```python
from build123d import *

# Parameters (mm, degrees)
SKETCH1_W                = 346
SKETCH1_H                = 134.5
BOSS_EXTRUDE1_DEPTH      = 6
M5_CLEARANCE_HOLE1_D     = 5.3
M5_CLEARANCE_HOLE2_D     = 5.3
SKETCH5_W                = 140
SKETCH5_H                = 70.4
CUT_EXTRUDE1_DEPTH       = 7
SKETCH6_R                = 10
BOSS_EXTRUDE2_DEPTH      = 6
FILLET1_R                = 5
M2_5_CLEARANCE_HOLE1_D   = 2.7
CUT_EXTRUDE29_DEPTH      = 7
SKETCH72_W               = 6.1
SKETCH72_H               = 10.1
CUT_EXTRUDE2_DEPTH       = 4
CUT_EXTRUDE2_DEPTH_BACK  = 4
SKETCH73_W               = 6.1
SKETCH73_H               = 10.1
CUT_EXTRUDE21_DEPTH      = 4
CUT_EXTRUDE21_DEPTH_BACK = 4
SKETCH74_W               = 6.1
SKETCH74_H               = 10.1
CUT_EXTRUDE22_DEPTH      = 4
CUT_EXTRUDE22_DEPTH_BACK = 4
SKETCH75_W               = 6.1
SKETCH75_H               = 10.1
CUT_EXTRUDE23_DEPTH      = 4
CUT_EXTRUDE23_DEPTH_BACK = 4
SKETCH76_W               = 6.1
SKETCH76_H               = 10.1
CUT_EXTRUDE24_DEPTH      = 4
CUT_EXTRUDE24_DEPTH_BACK = 4
SKETCH771_W              = 6.1
SKETCH771_H              = 10.1
CUT_EXTRUDE25_DEPTH      = 4
CUT_EXTRUDE25_DEPTH_BACK = 4
SKETCH781_W              = 6.1
SKETCH781_H              = 10.1
CUT_EXTRUDE26_DEPTH      = 4
CUT_EXTRUDE26_DEPTH_BACK = 4
SKETCH79_W               = 6.1
SKETCH79_H               = 10.1
CUT_EXTRUDE27_DEPTH      = 4
CUT_EXTRUDE27_DEPTH_BACK = 4
SKETCH710_W              = 6.1
SKETCH710_H              = 10.1
CUT_EXTRUDE28_DEPTH      = 4
CUT_EXTRUDE28_DEPTH_BACK = 4
SKETCH63_W               = 10
SKETCH63_H               = 6
CUT_EXTRUDE13_DEPTH      = 4
SKETCH64_W               = 10
SKETCH64_H               = 6
CUT_EXTRUDE14_DEPTH      = 4
M3_CLEARANCE_HOLE1_D     = 3.2
SKETCH786_W              = 16.25
SKETCH786_H              = 13.75
CUT_EXTRUDE30_DEPTH      = 7
M3_CLEARANCE_HOLE2_D     = 3.2
FILLET2_R                = 1
FILLET3_R                = 1


with BuildPart() as part:
    # Sketch1 → Boss-Extrude1 (new body)
    with BuildSketch(Plane(origin=(0, 0, 0), x_dir=(1, 0, 0), z_dir=(0, 1, 0))):
        Rectangle(SKETCH1_W, SKETCH1_H)
    extrude(amount=BOSS_EXTRUDE1_DEPTH)

    # M5 Clearance Hole1 (through all)
    with Locations(Plane(origin=(0, 6, 0), x_dir=(1, 0, 0), z_dir=(0, 1, 0))):
        with Locations((0, -61.25), (65, -61.25), (130, -61.25)):
            m5_clearance_hole1 = Hole(M5_CLEARANCE_HOLE1_D / 2)

    # Mirror1: M5 Clearance Hole1 across plane
    add(m5_clearance_hole1.mirror(Plane(origin=(0, 0, 0), x_dir=(0, 0, 1), z_dir=(1, 0, 0))), mode=Mode.SUBTRACT)

    # M5 Clearance Hole2 (through all)
    with Locations(Plane(origin=(0, 6, 0), x_dir=(1, 0, 0), z_dir=(0, 1, 0))):
        with Locations((166.4, -33.625), (166.4, 33.625)):
            m5_clearance_hole2 = Hole(M5_CLEARANCE_HOLE2_D / 2)

    # Mirror2: M5 Clearance Hole2 across plane
    add(m5_clearance_hole2.mirror(Plane(origin=(0, 0, 0), x_dir=(0, 0, 1), z_dir=(1, 0, 0))), mode=Mode.SUBTRACT)

    # Sketch5 → Cut-Extrude1 (cut, through all)
    with BuildSketch(Plane(origin=(0, 0, 0), x_dir=(-1, 0, 0), z_dir=(0, -1, 0))):
        with Locations((-78.4, -13.05)):
            Rectangle(SKETCH5_W, SKETCH5_H)
    extrude(amount=-CUT_EXTRUDE1_DEPTH, mode=Mode.SUBTRACT)

    # Sketch6 → Boss-Extrude2 (add)
    with BuildSketch(Plane.XZ):
        with Locations((8.4, -21.35)):
            Circle(SKETCH6_R)
        with Locations((8.4, 42.65)):
            Circle(SKETCH6_R)
        with Locations((146.4, -21.35)):
            Circle(SKETCH6_R)
    extrude(amount=-BOSS_EXTRUDE2_DEPTH)

    # Fillet1
    fillet1_edges = [part.edges().sort_by_distance(p)[0] for p in [
        (148.4, 3, -11.552041029),
        (148.4, 3, 48.25),
        (8.4, 3, -11.35),
        (18.367948636, 3, -22.15),
        (16.684926071, 3, 48.25),
        (8.4, 3, 32.65),
        (136.432051364, 3, -22.15),
    ]]
    fillet(fillet1_edges, radius=FILLET1_R)

    # M2.5 Clearance Hole1 (through all)
    with Locations(Plane(origin=(0, 6, 0), x_dir=(1, 0, 0), z_dir=(0, 1, 0))):
        with Locations((8.4, -42.65), (8.4, 21.35), (146.4, 21.35), (122.4, -52.65)):
            Hole(M2_5_CLEARANCE_HOLE1_D / 2)

    # Sketch783 → Cut-Extrude29 (cut, through all)
    with BuildSketch(Plane(origin=(0, 6, 0), x_dir=(1, 0, 0), z_dir=(0, 1, 0))):
        with BuildLine():
            Line((-76.023715784, 67.25), (-69.976284216, 67.25))
            ThreePointArc((-69.976284216, 67.25), (-70.5108067, 66.880601937), (-70.354248689, 66.25))
            ThreePointArc((-70.354248689, 66.25), (-73, 59.25), (-75.645751311, 66.25))
            ThreePointArc((-75.645751311, 66.25), (-75.4891933, 66.880601937), (-76.023715784, 67.25))
        make_face()
    cut_extrude29 = extrude(amount=-CUT_EXTRUDE29_DEPTH, mode=Mode.SUBTRACT)

    # Mirror4: Cut-Extrude29 across plane
    add(cut_extrude29.mirror(Plane.ZY.offset(-12)), mode=Mode.SUBTRACT)

    # Sketch72 → Cut-Extrude2 (cut, two sides)
    with BuildSketch(Plane(origin=(110, 3, 105.25), x_dir=(0, 0, -1), z_dir=(0, 1, 0))) as cut_extrude2_sk:
        with Locations((44, -32.5)):
            Rectangle(SKETCH72_W, SKETCH72_H)
        with Locations((44, -7.5)):
            Rectangle(SKETCH72_W, SKETCH72_H)
    extrude(amount=CUT_EXTRUDE2_DEPTH, mode=Mode.SUBTRACT)
    extrude(cut_extrude2_sk.sketch, amount=-CUT_EXTRUDE2_DEPTH_BACK, mode=Mode.SUBTRACT)

    # Sketch73 → Cut-Extrude21 (cut, two sides)
    with BuildSketch(Plane(origin=(45, 3, 105.25), x_dir=(0, 0, -1), z_dir=(0, 1, 0))) as cut_extrude21_sk:
        with Locations((44, -32.5)):
            Rectangle(SKETCH73_W, SKETCH73_H)
        with Locations((44, -7.5)):
            Rectangle(SKETCH73_W, SKETCH73_H)
    extrude(amount=CUT_EXTRUDE21_DEPTH, mode=Mode.SUBTRACT)
    extrude(cut_extrude21_sk.sketch, amount=-CUT_EXTRUDE21_DEPTH_BACK, mode=Mode.SUBTRACT)

    # Sketch74 → Cut-Extrude22 (cut, two sides)
    with BuildSketch(Plane(origin=(-20, 3, 105.25), x_dir=(0, 0, -1), z_dir=(0, 1, 0))) as cut_extrude22_sk:
        with Locations((44, -32.5)):
            Rectangle(SKETCH74_W, SKETCH74_H)
        with Locations((44, -7.5)):
            Rectangle(SKETCH74_W, SKETCH74_H)
    extrude(amount=CUT_EXTRUDE22_DEPTH, mode=Mode.SUBTRACT)
    extrude(cut_extrude22_sk.sketch, amount=-CUT_EXTRUDE22_DEPTH_BACK, mode=Mode.SUBTRACT)

    # Sketch75 → Cut-Extrude23 (cut, two sides)
    with BuildSketch(Plane(origin=(-85, 3, 105.25), x_dir=(0, 0, -1), z_dir=(0, 1, 0))) as cut_extrude23_sk:
        with Locations((44, -32.5)):
            Rectangle(SKETCH75_W, SKETCH75_H)
        with Locations((44, -7.5)):
            Rectangle(SKETCH75_W, SKETCH75_H)
    extrude(amount=CUT_EXTRUDE23_DEPTH, mode=Mode.SUBTRACT)
    extrude(cut_extrude23_sk.sketch, amount=-CUT_EXTRUDE23_DEPTH_BACK, mode=Mode.SUBTRACT)

    # Sketch76 → Cut-Extrude24 (cut, two sides)
    with BuildSketch(Plane(origin=(-150, 3, 105.25), x_dir=(0, 0, -1), z_dir=(0, 1, 0))) as cut_extrude24_sk:
        with Locations((44, -32.5)):
            Rectangle(SKETCH76_W, SKETCH76_H)
        with Locations((44, -7.5)):
            Rectangle(SKETCH76_W, SKETCH76_H)
    extrude(amount=CUT_EXTRUDE24_DEPTH, mode=Mode.SUBTRACT)
    extrude(cut_extrude24_sk.sketch, amount=-CUT_EXTRUDE24_DEPTH_BACK, mode=Mode.SUBTRACT)

    # Sketch771 → Cut-Extrude25 (cut, two sides)
    with BuildSketch(Plane(origin=(210.4, 3, 53.625), x_dir=(-1, 0, 0), z_dir=(0, 1, 0))) as cut_extrude25_sk:
        with Locations((44, -32.5)):
            Rectangle(SKETCH771_W, SKETCH771_H)
        with Locations((44, -7.5)):
            Rectangle(SKETCH771_W, SKETCH771_H)
    extrude(amount=CUT_EXTRUDE25_DEPTH, mode=Mode.SUBTRACT)
    extrude(cut_extrude25_sk.sketch, amount=-CUT_EXTRUDE25_DEPTH_BACK, mode=Mode.SUBTRACT)

    # Sketch781 → Cut-Extrude26 (cut, two sides)
    with BuildSketch(Plane(origin=(210.4, 3, -13.625), x_dir=(-1, 0, 0), z_dir=(0, 1, 0))) as cut_extrude26_sk:
        with Locations((44, -32.5)):
            Rectangle(SKETCH781_W, SKETCH781_H)
        with Locations((44, -7.5)):
            Rectangle(SKETCH781_W, SKETCH781_H)
    extrude(amount=CUT_EXTRUDE26_DEPTH, mode=Mode.SUBTRACT)
    extrude(cut_extrude26_sk.sketch, amount=-CUT_EXTRUDE26_DEPTH_BACK, mode=Mode.SUBTRACT)

    # Sketch79 → Cut-Extrude27 (cut, two sides)
    with BuildSketch(Plane(origin=(-122.4, 3, -13.625), x_dir=(-1, 0, 0), z_dir=(0, 1, 0))) as cut_extrude27_sk:
        with Locations((44, -32.5)):
            Rectangle(SKETCH79_W, SKETCH79_H)
        with Locations((44, -7.5)):
            Rectangle(SKETCH79_W, SKETCH79_H)
    extrude(amount=CUT_EXTRUDE27_DEPTH, mode=Mode.SUBTRACT)
    extrude(cut_extrude27_sk.sketch, amount=-CUT_EXTRUDE27_DEPTH_BACK, mode=Mode.SUBTRACT)

    # Sketch710 → Cut-Extrude28 (cut, two sides)
    with BuildSketch(Plane(origin=(-122.4, 3, 53.625), x_dir=(-1, 0, 0), z_dir=(0, 1, 0))) as cut_extrude28_sk:
        with Locations((44, -32.5)):
            Rectangle(SKETCH710_W, SKETCH710_H)
        with Locations((44, -7.5)):
            Rectangle(SKETCH710_W, SKETCH710_H)
    extrude(amount=CUT_EXTRUDE28_DEPTH, mode=Mode.SUBTRACT)
    extrude(cut_extrude28_sk.sketch, amount=-CUT_EXTRUDE28_DEPTH_BACK, mode=Mode.SUBTRACT)

    # Sketch63 → Cut-Extrude13 (cut, symmetric)
    with BuildSketch(Plane(origin=(47.5, 3, -59.242778608), x_dir=(0, 0, 1), z_dir=(0, 1, 0))):
        with Locations((0.767778608, -44)):
            Rectangle(SKETCH63_W, SKETCH63_H)
    cut_extrude13 = extrude(amount=CUT_EXTRUDE13_DEPTH, both=True, mode=Mode.SUBTRACT)

    # Sketch64 → Cut-Extrude14 (cut, symmetric)
    with BuildSketch(Plane(origin=(-40.5, 3, -40.157221392), x_dir=(0, 0, -1), z_dir=(0, 1, 0))):
        with Locations((0.767778608, -44)):
            Rectangle(SKETCH64_W, SKETCH64_H)
    cut_extrude14 = extrude(amount=CUT_EXTRUDE14_DEPTH, both=True, mode=Mode.SUBTRACT)

    # Mirror3: Cut-Extrude13, Cut-Extrude14 across plane
    add(cut_extrude13.mirror(Plane(origin=(12, 0, 0), x_dir=(0, 0, 1), z_dir=(1, 0, 0))), mode=Mode.SUBTRACT)
    add(cut_extrude14.mirror(Plane(origin=(12, 0, 0), x_dir=(0, 0, 1), z_dir=(1, 0, 0))), mode=Mode.SUBTRACT)

    # M3 Clearance Hole1 (through all)
    with Locations(Plane(origin=(0, 6, 0), x_dir=(1, 0, 0), z_dir=(0, 1, 0))):
        with Locations((-88, 59.75), (-58, 59.75), (82, 59.75), (112, 59.75)):
            Hole(M3_CLEARANCE_HOLE1_D / 2)

    # Sketch786 → Cut-Extrude30 (cut, through all)
    with BuildSketch(Plane.XZ):
        with Locations((-123, 28.25)):
            Rectangle(SKETCH786_W, SKETCH786_H)
    extrude(amount=-CUT_EXTRUDE30_DEPTH, mode=Mode.SUBTRACT)

    # M3 Clearance Hole2 (through all)
    with Locations(Plane(origin=(0, 0, 0), x_dir=(-1, 0, 0), z_dir=(0, -1, 0))):
        with Locations((108, -28.25), (138, -28.25)):
            Hole(M3_CLEARANCE_HOLE2_D / 2)

    # Fillet2
    fillet2_edges = [part.edges().sort_by_distance(p)[0] for p in [
        (-114.875, 3, 35.125),
        (-114.875, 3, 21.375),
        (-131.125, 3, 21.375),
        (-131.125, 3, 35.125),
    ]]
    fillet(fillet2_edges, radius=FILLET2_R)

    # Fillet3
    fillet3_edges = [part.edges().sort_by_distance(p)[0] for p in [
        (173, 3, 67.25),
        (-173, 3, 67.25),
        (-173, 3, -67.25),
        (173, 3, -67.25),
    ]]
    fillet(fillet3_edges, radius=FILLET3_R)


solid = part.part
```
Here's how the part is built. I have some questions about the finished solid (model axes, mm). Coordinates: 2 decimals unless noted, no trailing zeros. Order: outer loops, then holes, each group sorted by start corner. A loop starts at its lowest first (then second) coordinate and runs counter-clockwise, first axis right, second up.
Item 1: If we section it at B-B, the plane x = -144: List the corners of the cut face in (y, z) for me.
Response values:
outline: (0, -67.25) - (6, -67.25) - (6, 58.2) - (0, 58.2) - close; (0, 64.3) - (6, 64.3) - (6, 67.25) - (0, 67.25) - close
Item 2: I'm going to push flat-ended pins straight in: pin 1 Ø2.5 at (x, z) = (-58, -59.75) entering from +Y; pin 2 Ø3 at (x, z) = (8.4, 42.65) entering from +Y. Where does each tip first touch, or does it pass through?
Response values:
pin 1: passes through
pin 2: stops at y = 6
Item 3: If we section it at C-C, the plane y = 1.8: Give the number of separate pieces and of enclosed holes in the cut face, then the cut area to 3 significant figures.
Response values:
separate pieces: 1
enclosed holes: 43
area: 35,100 mm2
Item 4: Thinking about a two-plate mould opening in X: for faces 1 (the face through (-131.125, 3, 28)), 2 (the face through (-173, 3, 1)), which applies, pulls with the +X half, pulls with the -X half, needs draft (parallel to the pull), parting line crosses it, or undercut?
Response values:
face 1: undercut
face 2: pulls with the -X half
Item 5: If we section it at A-A, the plane z = 11: List the corners of the cut face in (x, y) for me.
Response values:
outline: (-173, 0) - (8.4, 0) - (8.4, 6) - (-173, 6) - close; (148.4, 0) - (173, 0) - (173, 6) - (148.4, 6) - close
Item 6: I need wall thicknesses on probe 1 along X at (y, z) = (1.25, 23.5) (3 decimals); probe 2 along X at (y, z) = (4.7, -44); probe 3 along X at (y, z) = (1.65, -18.5). Which ranges of each line are inside material? Lowest first, please.
Response values:
probe 1: x = -173 to -169.45, -163.35 to -131.125, -114.875 to 8.4, 148.4 to 163.35, 169.45 to 173
probe 2: x = -173 to -169.45, -163.35 to 0.5, 6.5 to 17.5, 23.5 to 163.35, 169.45 to 173
probe 3: x = -173 to -169.45, -163.35 to 17.99, 136.81 to 163.35, 169.45 to 173
